Read the model definition and answer for the solid it produces. Units are mm, in the model's axes. A direction names the side the tool comes from. Coordinates: 2 decimals unless noted, no trailing zeros. Order: outer loops, then holes, each group sorted by start corner. A loop starts at its lowest first (then second) coordinate and runs counter-clockwise, first axis right, second up. Notation, with made-up numbers: (-16.75, -17) -> (12.25, -17) arc R32 ccw to (12.25, 10) -> close; hole circle Ø3 at (0, 57.5). An arc over 180 degrees is marked (long way). Answer as a JSON object with one key per item and string values. Group by question number.
1) Section A-A on z = 0 is taken. Determine the outline of the cut face in (x, y), and give its area (3 significant figures).
2) Section D-D on x = -18.5 is taken. Determine the outline of the cut face in (y, z), and give its area (3 significant figures).
3) Section C-C on y = 26.75 is taken. Determine the outline of the cut face in (x, z), and give its area (3 significant figures).
4) Determine the mould class of faces 1 (the cylindrical face through (28.38, 1.97, -54.56)), 2 (the flat face through (26, 20, 9)), 3 (the flat face through (13, 0, 1)) for opening direction Z: released by +Z, released by -Z, zero draft, split by the parting line, or undercut.
5) Consider L1, parallel to X at y = 22.25, z = 0; L2, parallel to Z at x = 40, y = 13.75; L3, parallel to Z at x = -37.5, y = 29. Determine where each line is inside the solid, lowest interval first.
6) A tool of negligible diameter and unlimited length cuts with its end or side. For faces 4 (the cylindrical face through (-43, 15, 0)), 5 (the flat face through (30, 20, 41.5)), 6 (the flat face through (29, 20, 12)), from which of +Z, -Z, +X, -X, +Y, -Y can it reach the whole face along a straight path? Write none if from no direction.
7) Given pin 1 (10 mm diameter, centred on x = 19, y = 9.5, fed in from +Z); pin 2 (1 mm diameter, centred on y = 23.5, z = 33, fed in from -X); pin 3 (1.8 mm diameter, centred on y = 18, z = 14.5, fed in from -X), each flat-ended and moving along its own axis, determine where each tip first touches the part or whether it passes through.
8) Section B-B on x = 0 is taken. Determine the outline of the cut face in (y, z).
from build123d import *

# Parameters (mm, degrees)
ESQUISSE1_R             = 3
ESQUISSE1_W             = 25
ESQUISSE1_H             = 11
BOSS_EXTRU_1_DEPTH      = 30
ESQUISSE2_R             = 125
ESQUISSE2_R_2           = 53.5
ENL_V_MAT_EXTRU_1_DEPTH = 31
ESQUISSE8_R             = 61.5
ESQUISSE8_R_2           = 53.5
BOSS_EXTRU_2_DEPTH      = 4
ESQUISSE5_R             = 18
ENL_V_MAT_EXTRU_2_DEPTH = 11
ESQUISSE6_W             = 41
ESQUISSE6_H             = 39
ESQUISSE6_W_2           = 7
ESQUISSE6_H_2           = 6
ESQUISSE6_W_3           = 17
ESQUISSE6_H_3           = 8
ENL_V_MAT_EXTRU_3_DEPTH = 21
ESQUISSE7_W             = 36
ESQUISSE7_H             = 11
ENL_V_MAT_EXTRU_4_DEPTH = 11


with BuildPart() as part:
    # Esquisse1 → Boss.-Extru.1 (new body)
    with BuildSketch(Plane(origin=(0, 0, 0), x_dir=(1, 0, 0), z_dir=(0, 1, 0))):
        with BuildLine():
            ThreePointArc((68.106918153, 104.816256848), (54.23546739, 112.621108488), (39.484680574, 118.6))
            ThreePointArc((39.484680574, 118.6), (0, 85), (-39.484680574, 118.6))
            ThreePointArc((-39.484680574, 118.6), (-54.23546739, 112.621108488), (-68.106918153, 104.816256848))
            ThreePointArc((-68.106918153, 104.816256848), (-66.45567601, 52.996633158), (-117.343509488, 43.075524153))
            ThreePointArc((-117.343509488, 43.075524153), (-121.865989023, 27.815116745), (-124.412618383, 12.103734428))
            ThreePointArc((-124.412618383, 12.103734428), (-82.868872535, -18.914279386), (-106.840282387, -64.885699962))
            ThreePointArc((-106.840282387, -64.885699962), (-97.728935309, -77.936225232), (-87.033079415, -89.723146888))
            ThreePointArc((-87.033079415, -89.723146888), (-36.880117825, -76.582353772), (-15.884143503, -123.986668578))
            ThreePointArc((-15.884143503, -123.986668578), (0, -125), (15.884143503, -123.986668578))
            ThreePointArc((15.884143503, -123.986668578), (36.880117825, -76.582353772), (87.033079415, -89.723146888))
            ThreePointArc((87.033079415, -89.723146888), (97.728935309, -77.936225232), (106.840282387, -64.885699962))
            ThreePointArc((106.840282387, -64.885699962), (82.868872535, -18.914279386), (124.412618383, 12.103734428))
            ThreePointArc((124.412618383, 12.103734428), (121.865989023, 27.815116745), (117.343509488, 43.075524153))
            ThreePointArc((117.343509488, 43.075524153), (66.45567601, 52.996633158), (68.106918153, 104.816256848))
        make_face()
        with Locations((-40, 0)):
            Circle(ESQUISSE1_R, mode=Mode.SUBTRACT)
        with Locations((40, 0)):
            Circle(ESQUISSE1_R, mode=Mode.SUBTRACT)
        Rectangle(ESQUISSE1_W, ESQUISSE1_H, mode=Mode.SUBTRACT)
    extrude(amount=BOSS_EXTRU_1_DEPTH)

    # Esquisse2 → Enlèv. mat.-Extru.1 (cut, through all)
    with BuildSketch(Plane(origin=(0, 30, 0), x_dir=(1, 0, 0), z_dir=(0, 1, 0))):
        Circle(ESQUISSE2_R)
        Circle(ESQUISSE2_R_2, mode=Mode.SUBTRACT)
    extrude(amount=-ENL_V_MAT_EXTRU_1_DEPTH, mode=Mode.SUBTRACT)

    # Esquisse8 → Boss.-Extru.2 (add)
    with BuildSketch(Plane.XZ):
        Circle(ESQUISSE8_R)
        Circle(ESQUISSE8_R_2, mode=Mode.SUBTRACT)
    extrude(amount=-BOSS_EXTRU_2_DEPTH)

    # Esquisse5 → Enlèv. mat.-Extru.2 (cut)
    with BuildSketch(Plane(origin=(0, 0, 5.5), x_dir=(-1, 0, 0), z_dir=(0, 0, -1))):
        with Locations((-16, 19)):
            Circle(ESQUISSE5_R)
    extrude(amount=ENL_V_MAT_EXTRU_2_DEPTH, mode=Mode.SUBTRACT)

    # Esquisse6 → Enlèv. mat.-Extru.3 (cut)
    with BuildSketch(Plane(origin=(0, 30, 0), x_dir=(1, 0, 0), z_dir=(0, 1, 0))):
        with Locations((5.5, -25)):
            Rectangle(ESQUISSE6_W, ESQUISSE6_H)
        with Locations((-18.5, -15)):
            Rectangle(ESQUISSE6_W_2, ESQUISSE6_H_2)
        with Locations((29.5, -15)):
            Rectangle(ESQUISSE6_W_2, ESQUISSE6_H_2)
        with Locations((34.5, -37.5)):
            Rectangle(ESQUISSE6_W_3, ESQUISSE6_H_3)
    extrude(amount=-ENL_V_MAT_EXTRU_3_DEPTH, mode=Mode.SUBTRACT)

    # Esquisse7 → Enlèv. mat.-Extru.4 (cut)
    with BuildSketch(Plane(origin=(0, 30, 0), x_dir=(1, 0, 0), z_dir=(0, 1, 0))):
        with Locations((16, 0)):
            Rectangle(ESQUISSE7_W, ESQUISSE7_H)
    extrude(amount=-ENL_V_MAT_EXTRU_4_DEPTH, mode=Mode.SUBTRACT)


solid = part.part
Worked answers:
{
 "1": {"outline": "(-61.5, 0) -> (-43, 0) -> (-43, 30) -> (-53.5, 30) -> (-53.5, 4) -> (-61.5, 4) -> close; (-37, 0) -> (-12.5, 0) -> (-12.5, 30) -> (-37, 30) -> close; (12.5, 0) -> (37, 0) -> (37, 30) -> (34, 30) -> (34, 19) arc R18 cw to (12.5, 1.34) -> close; (43, 0) -> (61.5, 0) -> (61.5, 4) -> (53.5, 4) -> (53.5, 30) -> (43, 30) -> close", "area": "1,610 mm²"},
 "2": {"outline": "(0, -58.65) -> (4, -58.65) -> (4, -50.2) -> (30, -50.2) -> (30, 12) -> (9, 12) -> (9, 18) -> (30, 18) -> (30, 50.2) -> (4, 50.2) -> (4, 58.65) -> (0, 58.65) -> close", "area": "2,950 mm²"},
 "3": {"outline": "(-22, 12) -> (-22, 18) -> (-15, 18) -> (-15, 44.5) -> (26, 44.5) -> (26, 41.5) -> (33.76, 41.5) arc R53.5 ccw (long way) to (41.71, 33.5) -> (26, 33.5) -> (26, 18) -> (33, 18) -> (33, 12) -> (26, 12) -> (26, 5.5) -> (34, 5.5) -> (34, -5.5) -> (-12.5, -5.5) -> (-12.5, 5.5) -> (-15, 5.5) -> (-15, 12) -> close; hole circle Ø6 at (-40, 0); hole circle Ø6 at (40, 0)", "area": "6,640 mm²"},
 "4": {"face 1": "split by the parting line", "face 2": "undercut", "face 3": "zero draft"},
 "5": {"L1": "x = -53.5 to -43, -37 to -12.5, 34 to 37, 43 to 53.5", "L2": "z = -35.53 to -3, 3 to 33.5", "L3": "z = -38.16 to -1.66, 1.66 to 38.16"},
 "6": {"face 4": "+Y, -Y", "face 5": "+X, +Y", "face 6": "+Y"},
 "7": {"pin 1": "stops at z = 51.64", "pin 2": "stops at x = -42.5", "pin 3": "stops at x = -51.74"},
 "8": {"outline": "(0, -61.5) -> (4, -61.5) -> (4, -53.5) -> (30, -53.5) -> (30, -5.5) -> (0, -5.5) -> close; (0, 5.5) -> (9, 5.5) -> (9, 44.5) -> (30, 44.5) -> (30, 53.5) -> (4, 53.5) -> (4, 61.5) -> (0, 61.5) -> close"}
}
